Input: part model. Units: mm. Frame: model coordinates. A direction names the side the tool comes from. Coordinates: 2 decimals unless noted, no trailing zeros. Write each loop counter-clockwise with the first axis right and the second up, starting at its lowest first coordinate (ties: lowest second). Pieces come first, ordered by that corner, then holes. Notation, with made-up numbers: (67, 70.5) - (77, 70.5) arc R24 cw to (77, 106.5) - close; hole circle Ø10 at (-1.75, 56.5). An arc over 180 degrees is marked (long way). One line per question, with ' | ' between items. Start each with the question number.
1) Section query D-D on x = 0.25. Return loops of the section in (y, z), and give its area (3 significant figures).
2) Reachability of faces 4 (the flat face through (-2.46, -1, 0)), 5 (the flat face through (-1.953, -0.986, -5.01)), 6 (the flat face through (7, 0.2, 7.5)) from +Z, -Z, +X, -X, +Y, -Y: full face, straight path, thin tool, end or side. Return the list, or none.
3) Line query: line 1 (X direction, y = 1.65, z = 1.5); line 2 (Z direction, x = -0.25, y = 0.9); line 3 (X direction, y = -0.9, z = -0.75). Output: solid intervals per line, ascending.
4) Draft query along X for faces 1 (the cylindrical face through (-0.014, 3.715, 7.699)), 2 (the flat face through (1.967, -1.014, 5.01)), 3 (the cylindrical face through (1.715, 2.754, -7.699)). Return one class per face: released by +X, released by -X, zero draft, split by the parting line, or undercut.
5) Section query C-C on y = -0.3. Return loops of the section in (x, z), and give its area (3 significant figures).
6) Section query A-A on z = 4.75. Return loops of the section in (x, y).
7) First-contact query: P1, Ø0.6, axis at y = 3, z = -6.5, coming from the +X side; P2, Ø3.5, axis at x = -2.5, z = -0.5, coming from the +Y side. Flat tips, straight axial feed; report the tip coordinate or a pass-through.
8) Section query B-B on x = 3.25. Return loops of the section in (y, z).
```python
from build123d import *

# Parameters (mm, degrees)
SKETCH1_W           = 16
SKETCH1_H           = 17
SKETCH1_W_2         = 11
SKETCH1_H_2         = 12
BOSS_EXTRUDE1_DEPTH = 2.5
SKETCH2_W           = 16
SKETCH2_H           = 17
BOSS_EXTRUDE2_DEPTH = 2
SKETCH4_W           = 2.7
SKETCH4_H           = 11.5
CUT_EXTRUDE1_DEPTH  = 12.937336386
CHAMFER1_SIZE       = 2
SKETCH5_W           = 4
SKETCH5_H           = 2
BOSS_EXTRUDE3_DEPTH = 1.5
FILLET1_R           = 1
FILLET2_R           = 1
CUT_EXTRUDE2_DEPTH  = 1.5
CUT_EXTRUDE3_DEPTH  = 1.5


with BuildPart() as part:
    # Sketch1 → Boss-Extrude1 (new body)
    with BuildSketch(Plane(origin=(0, 0, 0), x_dir=(1, 0, 0), z_dir=(0, 1, 0))):
        Rectangle(SKETCH1_W, SKETCH1_H)
        Rectangle(SKETCH1_W_2, SKETCH1_H_2, mode=Mode.SUBTRACT)
    extrude(amount=BOSS_EXTRUDE1_DEPTH)

    # Sketch2 → Boss-Extrude2 (add)
    with BuildSketch(Plane.XZ):
        Rectangle(SKETCH2_W, SKETCH2_H)
    extrude(amount=BOSS_EXTRUDE2_DEPTH)

    # Sketch4 → Cut-Extrude1 (cut, through all)
    with BuildSketch(Plane(origin=(0, 0, 0), x_dir=(1, 0, 0), z_dir=(0, 1, 0))):
        with Locations((-3.81, 0)):
            Rectangle(SKETCH4_W, SKETCH4_H)
        with Locations((3.81, 0)):
            Rectangle(SKETCH4_W, SKETCH4_H)
    extrude(amount=-CUT_EXTRUDE1_DEPTH, mode=Mode.SUBTRACT)

    # Chamfer1
    chamfer1_edges = [part.edges().sort_by_distance(p)[0] for p in [
        (-8, 0.25, -8.5),
        (8, 0.25, -8.5),
        (8, 0.25, 8.5),
        (-8, 0.25, 8.5),
    ]]
    chamfer(chamfer1_edges, length=CHAMFER1_SIZE)

    # Sketch5 → Boss-Extrude3 (add)
    with BuildSketch(Plane(origin=(0, 2.5, 0), x_dir=(1, 0, 0), z_dir=(0, 1, 0))):
        with Locations((0, 7)):
            Rectangle(SKETCH5_W, SKETCH5_H)
        with Locations((0, -7)):
            Rectangle(SKETCH5_W, SKETCH5_H)
    extrude(amount=BOSS_EXTRUDE3_DEPTH)

    # Fillet1
    fillet1_edges = [part.edges().sort_by_distance(p)[0] for p in [
        (2, 4, -7),
        (-2, 4, -7),
        (2, 4, 7),
        (-2, 4, 7),
    ]]
    fillet(fillet1_edges, radius=FILLET1_R)

    # Fillet2
    fillet2_edges = [part.edges().sort_by_distance(p)[0] for p in [
        (2, 2.75, -8),
        (0, 4, -8),
        (-2, 2.75, -8),
        (-1.707106781, 3.707106781, -8),
        (1.707106781, 3.707106781, -8),
        (2, 2.75, 8),
        (0, 4, 8),
        (-2, 2.75, 8),
        (-1.707106781, 3.707106781, 8),
        (1.707106781, 3.707106781, 8),
    ]]
    fillet(fillet2_edges, radius=FILLET2_R)

    # Sketch6 → Cut-Extrude2 (cut)
    with BuildSketch(Plane.XY.offset(-5.75)):
        Polygon((-2.46, -2), (-2.46, 0), (-1.46, 0), align=None)
        Polygon((2.46, -2), (2.46, 0), (1.46, 0), align=None)
    extrude(amount=CUT_EXTRUDE2_DEPTH, mode=Mode.SUBTRACT)

    # Sketch8 → Cut-Extrude3 (cut)
    with BuildSketch(Plane(origin=(0, 0, 5.75), x_dir=(-1, 0, 0), z_dir=(0, 0, -1))):
        Polygon((-2.46, 0), (-2.46, -2), (-1.46, 0), align=None)
        Polygon((2.46, -2), (2.46, 0), (1.46, 0), align=None)
    extrude(amount=CUT_EXTRUDE3_DEPTH, mode=Mode.SUBTRACT)


solid = part.part
```
Answer key:
1) outline: (-2, -8.5) - (2.5, -8.5) - (2.5, -8) - (3, -8) arc R1 ccw to (4, -7) - (4, -6) - (0, -6) - (0, 6) - (4, 6) - (4, 7) arc R1 ccw to (3, 8) - (2.5, 8) - (2.5, 8.5) - (-2, 8.5) - close | area: 52.1 mm²
2) face 4: +Y, -Y | face 5: +Y | face 6: +Z, +X, +Y, -Y
3) line 1: -8 to -5.5, 5.5 to 8 | line 2: -8.5 to -6, 6 to 8.5 | line 3: -8 to -5.16, -2.46 to 2.46, 5.16 to 8
4) face 1: zero draft | face 2: undercut | face 3: released by +X
5) outline: (-8, -6.5) - (-6, -8.5) - (6, -8.5) - (8, -6.5) - (8, 6.5) - (6, 8.5) - (-6, 8.5) - (-8, 6.5) - close; hole (-5.16, -5.75) - (-1.61, -5.75) - (-1.61, -4.25) - (-2.46, -4.25) - (-2.46, 4.25) - (-1.61, 4.25) - (-1.61, 5.75) - (-5.16, 5.75) - close; hole (1.61, -5.75) - (5.16, -5.75) - (5.16, 5.75) - (1.61, 5.75) - (1.61, 4.25) - (2.46, 4.25) - (2.46, -4.25) - (1.61, -4.25) - close | area: 197 mm²
6) outline: (-8, -2) - (-5.16, -2) - (-5.16, 0) - (-5.5, 0) - (-5.5, 2.5) - (-8, 2.5) - close; (-2.46, -2) - (2.46, -2) - (1.46, 0) - (-1.46, 0) - close; (5.16, -2) - (8, -2) - (8, 2.5) - (5.5, 2.5) - (5.5, 0) - (5.16, 0) - close
7) P1: x = 2 | P2: y = 0
8) outline: (-2, -8.5) - (2.5, -8.5) - (2.5, -6) - (0, -6) - (0, -5.75) - (-2, -5.75) - close; (-2, 5.75) - (0, 5.75) - (0, 6) - (2.5, 6) - (2.5, 8.5) - (-2, 8.5) - close
